Input: part model. Units: mm. Frame: model coordinates. A direction names the side the tool comes from. Coordinates: 2 decimals unless noted, no trailing zeros. Order: outer loops, then holes, each group sorted by start corner. A loop starts at its lowest first (then second) coordinate and runs counter-clockwise, first axis right, second up. Notation, with made-up numbers: (-36.5, 70.25) -> (-23.5, 70.25) arc R9 ccw to (-23.5, 80.25) -> close; hole circle Ø9 at (-11, -18.75). An arc over 180 degrees is marked (long way). Use CSV: the item, a comma, the result in double quotes. Start each with the question number.
```python
from build123d import *

# Parameters (mm, degrees)
SKETCH_R        = 11.45
SKETCH_R_2      = 8.45
PAD_DEPTH       = 3
SKETCH001_R     = 11.45
SKETCH001_R_2   = 7.125
PAD001_DEPTH    = 6.5
CHAMFER_SIZE    = 0.7
CHAMFER001_SIZE = 1


with BuildPart() as part:
    # Sketch → Pad (new body)
    with BuildSketch(Plane.XY):
        Circle(SKETCH_R)
        Circle(SKETCH_R_2, mode=Mode.SUBTRACT)
    extrude(amount=PAD_DEPTH)

    # Sketch001 (on Face4 of Pad) → Pad001 (join)
    with BuildSketch(Plane.XY.offset(3)):
        Circle(SKETCH001_R)
        Circle(SKETCH001_R_2, mode=Mode.SUBTRACT)
    extrude(amount=PAD001_DEPTH)

    # Chamfer
    chamfer_edges = [part.edges().sort_by_distance(p)[0] for p in [
        (-8.45, 0, 0),
    ]]
    chamfer(chamfer_edges, length=CHAMFER_SIZE)

    # Chamfer001
    chamfer001_edges = [part.edges().sort_by_distance(p)[0] for p in [
        (-7.125, 0, 9.5),
    ]]
    chamfer(chamfer001_edges, length=CHAMFER001_SIZE)


solid = part.part
```
1. Section C-C on z = 7.75. Return loops of the section in (x, y) (3 decimals).
2. Contact query for flat-ended pins moving along their axis: P1, Ø2, axis at x = 4.5, y = 4.5, coming from the -Z side; P2, Ø13.5, axis at x = -1, y = -3, coming from the -Z side; P3, Ø1.5, axis at y = -6.5, z = 8.5, coming from the -X side. Output: stop coordinate, or through.
3. Section A-A on y = 0. Return loops of the section in (x, z) (3 decimals).
4. Material intervals for line 1 along Y through (x, z) = (0.25, 6.5); line 2 along Y through (x, z) = (0, 2.3), sorted ascending.
5. Access query for faces 1 (the face through (-2.48, -11.18, 4.68)), 2 (the face through (8.06, 2.54, 1.83)). Directions: +Z, -Z, +X, -X, +Y, -Y. A direction counts if a zero-diameter tool reaches every point of the face in a straight line with its end or side. Return the directions, or none.
6. Section D-D on z = 2.5. Return loops of the section in (x, y), then the cut area to 3 significant figures.
Values follow:
1,outline,"circle Ø22.9 at (0, 0); hole circle Ø14.25 at (0, 0)"
2,P1,"stops at z = 3"
2,P2,"stops at z = 0"
2,P3,"stops at x = -9.9"
3,outline,"(-11.45, 0) -> (-9.15, 0) -> (-8.45, 0.7) -> (-8.45, 3) -> (-7.125, 3) -> (-7.125, 8.5) -> (-8.125, 9.5) -> (-11.45, 9.5) -> close; (7.125, 3) -> (8.45, 3) -> (8.45, 0.7) -> (9.15, 0) -> (11.45, 0) -> (11.45, 9.5) -> (8.125, 9.5) -> (7.125, 8.5) -> close"
4,line 1,"y = -11.45 to -7.12, 7.12 to 11.45"
4,line 2,"y = -11.45 to -8.45, 8.45 to 11.45"
5,face 1,"+Z, -Z"
5,face 2,"-Z"
6,outline,"circle Ø22.9 at (0, 0); hole circle Ø16.9 at (0, 0)"
6,area,"188 mm2"
